Here's how the part is built. I have some questions about the finished solid (model axes, mm). Face numbers are marked on the shaded views. Round coordinates to 2 decimals unless told otherwise and drop trailing zeros. Write each loop counter-clockwise with the first axis right and the second up, starting at its lowest first coordinate (ties: lowest second). Pieces come first, ordered by that corner, then holes. Notation, with made-up numbers: (71, -1.75) -> (90, -1.75) arc R16 cw to (90, 6.25) -> close; hole circle Ø4 at (-39.75, 15.25). An arc over 180 degrees is marked (long way). Put each result on its own line as item: value. Start each with the question number.
1. Suppose I cut it at B-B (z = 83). Please give me the cut outline in (x, y), then the cut area to 3 significant figures.
2. I need wall thicknesses on probe 1 along Z at (x, y) = (27, 31); probe 2 along Y at (x, z) = (70.5, 56); probe 3 along X at (y, z) = (-7.5, 93.5). Which ranges of each line are inside material? Lowest first, please. Write a range as from..to.
3. For pin 1 (8 mm diameter, centred on x = 14, z = 69, fed in from -Y); pin 2 (1 mm diameter, centred on y = 31.5, z = 35, fed in from +X); pin 3 (12 mm diameter, centred on y = 3.5, z = 45.5, fed in from +X); pin 4 (2.5 mm diameter, centred on x = 18.69, y = 27.96, fed in from -Z), each with a flat end and sliding along its axis, tell me the tip position at first contact or that it passes through.
4. We'd pull the mould along X, two halves only. Please class the marked faces 1, 2 and 3: +X half, -X half, draft (parallel to the pull), parting line (faces both ways), or undercut.
5. Suppose I cut it at A-A (y = 11). Please give me the cut outline in (x, z), then the cut area to 3 significant figures.
6. Suppose I cut it at C-C (x = 37). Please give me the cut outline in (y, z).
```python
from build123d import *

# Parameters (mm, degrees)
EXTRUDE_1_DEPTH           = 3
EXTRUDE_2_DEPTH           = 104
EXTRUDE_3_DEPTH           = 3
CUT_EXTRUDE_1_DEPTH       = 159.483205287
HOLE_WIZARD_3_0_3_1_D     = 3
HOLE_WIZARD_3_0_3_1_DEPTH = 3
HOLE_WIZARD_3_0_3_2_D     = 3
HOLE_WIZARD_3_0_3_2_DEPTH = 110


with BuildPart() as part:
    # 草图1 → 凸台-拉伸1 (new body)
    with BuildSketch(Plane.XY.offset(110)):
        with BuildLine():
            Line((48.043658488, 49.686561818), (16.083624337, 44.189394688))
            Line((16.083624337, 44.189394688), (0, 0))
            ThreePointArc((0, 0), (49.31823123, -22.233763367), (103.260442774, -18.126942356))
            Line((103.260442774, -18.126942356), (81.890470472, 43.311728011))
            add(Edge.make_bspline(
                [(48.043658488, 49.686561818), (60.031404168, 34.166493651), (81.890470472, 43.311728011)],
                knots=[3.390052137, 3.390052137, 3.390052137, 4.76191312, 4.76191312, 4.76191312], degree=2, weights=[1, 0.773830015, 1]))
        make_face()
    extrude(amount=-EXTRUDE_1_DEPTH)

    # 草图2 → 凸台-拉伸2 (add)
    with BuildSketch(Plane(origin=(0, 0, 107), x_dir=(-1, 0, 0), z_dir=(0, 0, -1))):
        with BuildLine():
            Line((-3.564517285, 1.022017551), (-19.489368658, 44.775187108))
            Line((-19.489368658, 44.775187108), (-16.083624337, 44.189394688))
            Line((-16.083624337, 44.189394688), (0, 0))
            ThreePointArc((0, 0), (-49.31823123, -22.233763367), (-103.260442774, -18.126942356))
            Line((-103.260442774, -18.126942356), (-102.274839972, -15.293334302))
            ThreePointArc((-102.274839972, -15.293334302), (-50.883106444, -19.457225166), (-3.564517285, 1.022017551))
        make_face()
    extrude(amount=EXTRUDE_2_DEPTH)

    # 草图3 → 凸台-拉伸3 (add)
    with BuildSketch(Plane(origin=(0, 0, 3), x_dir=(-1, 0, 0), z_dir=(0, 0, -1))):
        with BuildLine():
            Line((-77.887672968, 54.819770834), (-16.083624337, 44.189394688))
            Line((-16.083624337, 44.189394688), (0, 0))
            ThreePointArc((0, 0), (-49.31823123, -22.233763367), (-103.260442774, -18.126942356))
            Line((-103.260442774, -18.126942356), (-77.887672968, 54.819770834))
        make_face()
    extrude(amount=EXTRUDE_3_DEPTH)

    # 草图4 → 切除-拉伸1 (cut, through all)
    with BuildSketch(Plane.XY.offset(3)):
        with BuildLine():
            Line((77.887672968, 54.819770834), (48.043658488, 49.686561818))
            add(Edge.make_bspline(
                [(48.043658488, 49.686561818), (60.032354081, 34.167172902), (81.890470472, 43.311728011)],
                knots=[3.389784889, 3.389784889, 3.389784889, 4.7613973, 4.7613973, 4.7613973], degree=2, weights=[1, 0.773908731, 1]))
            Line((81.890470472, 43.311728011), (77.887672968, 54.819770834))
        make_face()
    extrude(amount=-CUT_EXTRUDE_1_DEPTH, mode=Mode.SUBTRACT)

    # Ø3.0 (3) 直径孔1
    with Locations(Plane(origin=(0, 0, 107), x_dir=(-1, 0, 0), z_dir=(0, 0, -1))):
        with Locations((-18.688258909, 27.955134161), (-23.158328606, 39.628543128)):
            Hole(HOLE_WIZARD_3_0_3_1_D / 2, depth=HOLE_WIZARD_3_0_3_1_DEPTH)

    # Ø3.0 (3) 直径孔2
    with Locations(Plane(origin=(0, 0, 0), x_dir=(-1, 0, 0), z_dir=(0, 0, -1))):
        with Locations((-18.688258909, 27.955134161), (-23.158328606, 39.628543128)):
            Hole(HOLE_WIZARD_3_0_3_2_D / 2, depth=HOLE_WIZARD_3_0_3_2_DEPTH)


solid = part.part
```
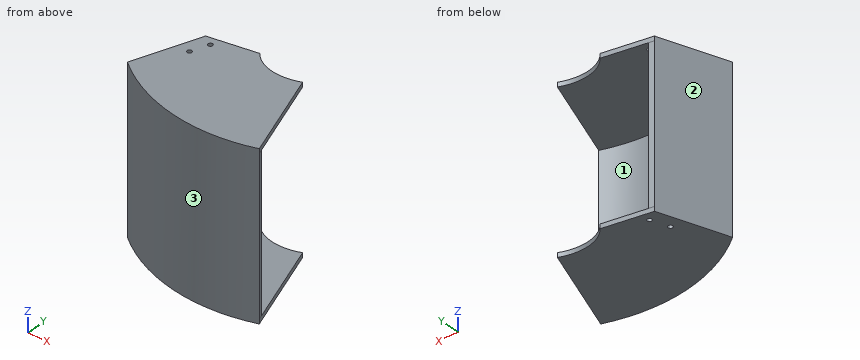
Verdict:
1. outline: (0, 0) arc R109.43 ccw to (103.26, -18.13) -> (102.27, -15.29) arc R106.43 cw to (3.56, 1.02) -> (19.49, 44.78) -> (16.08, 44.19) -> close
1. area: 461 mm^2
2. probe 1: z = 0..3, 107..110
2. probe 2: y = -23.86..-20.86
2. probe 3: x = 10.65..16.57
3. pin 1: stops at y = -11.67
3. pin 2: stops at x = 14.84
3. pin 3: stops at x = 8.45
3. pin 4: passes through
4. face 1: undercut
4. face 2: -X half
4. face 3: parting line
5. outline: (4, 0) -> (93.13, 0) -> (93.13, 3) -> (7.2, 3) -> (7.2, 107) -> (93.13, 107) -> (93.13, 110) -> (4, 110) -> close
5. area: 867 mm^2
6. outline: (-19.33, 0) -> (47.79, 0) -> (47.79, 3) -> (-16.19, 3) -> (-16.19, 107) -> (47.79, 107) -> (47.79, 110) -> (-19.33, 110) -> close
